Can you work these out from the model? Positions are in its coordinate system, mm. A direction names the side the tool comes from. Round coordinates to 2 decimals unless told otherwise and drop trailing zeros. Write each loop counter-clockwise with the first axis right and the second up, starting at its lowest first coordinate (ties: lowest second). Pieces come first, ordered by that corner, then holes. Notation, with made-up numbers: (32.5, 19) -> (40.5, 19) arc R23 ccw to (40.5, 45) -> close; hole circle Ø8 at (26, -16). An arc over 180 degrees is marked (long way). Use CSV: the item, a comma, the result in double quotes.
```python
from build123d import *

# Parameters (mm, degrees)
SKETCH1_W                = 150.2
SKETCH1_H                = 64
BOSS_EXTRUDE1_DEPTH      = 6
FILLET1_R                = 5
BOSS_EXTRUDE2_DEPTH      = 40
BOSS_EXTRUDE2_DEPTH_BACK = 10
SKETCH2_W                = 60
SKETCH2_H                = 6
FILLET2_R                = 5
SKETCH3_R                = 40
BOSS_EXTRUDE4_DEPTH      = 6
FILLET4_R                = 5
SKETCH4_R                = 1.55
CUT_EXTRUDE1_DEPTH       = 167.673453195
CUT_EXTRUDE2_START       = -10
CUT_EXTRUDE2_DEPTH       = 10
FILLET5_R                = 5
SKETCH6_R                = 1.5
CUT_EXTRUDE3_DEPTH       = 167.673453195
SKETCH7_R                = 1.5
CUT_EXTRUDE4_DEPTH       = 167.673453195
SKETCH9_R                = 3.2
CUT_EXTRUDE5_DEPTH       = 3


with BuildPart() as part:
    # Sketch1 → Boss-Extrude1 (new body)
    with BuildSketch(Plane.XY):
        with Locations((75.1, 32)):
            Rectangle(SKETCH1_W, SKETCH1_H)
    extrude(amount=BOSS_EXTRUDE1_DEPTH)

    # Fillet1
    fillet1_edges = [part.edges().sort_by_distance(p)[0] for p in [
        (0, 64, 3),
        (150.2, 64, 3),
        (150.2, 0, 3),
        (0, 0, 3),
    ]]
    fillet(fillet1_edges, radius=FILLET1_R)

    # Sketch2 → Boss-Extrude2 (add, two sides: drawn at the far end of the back side and taken through both)
    with BuildSketch(Plane.XZ.offset(-BOSS_EXTRUDE2_DEPTH_BACK)):
        with Locations((30, 3)):
            Rectangle(SKETCH2_W, SKETCH2_H)
    extrude(amount=BOSS_EXTRUDE2_DEPTH + BOSS_EXTRUDE2_DEPTH_BACK)

    # Fillet2
    fillet2_edges = [part.edges().sort_by_distance(p)[0] for p in [
        (0, -40, 3),
        (60, -40, 3),
    ]]
    fillet(fillet2_edges, radius=FILLET2_R)

    # Sketch3 → Boss-Extrude4 (add)
    with BuildSketch(Plane.XY.offset(6)):
        with Locations((75.1, 32)):
            Circle(SKETCH3_R)
    extrude(amount=-BOSS_EXTRUDE4_DEPTH)

    # Fillet4
    fillet4_edges = [part.edges().sort_by_distance(p)[0] for p in [
        (60, -5.040383367, 3),
        (99.1, 0, 3),
        (99.1, 64, 3),
        (51.1, 64, 3),
    ]]
    fillet(fillet4_edges, radius=FILLET4_R)

    # Sketch4 → Cut-Extrude1 (cut, through all)
    with BuildSketch(Plane.XY.offset(6)):
        with Locations((75.1, 41.525)):
            Circle(SKETCH4_R)
        with Locations((83.348891971, 36.7625)):
            Circle(SKETCH4_R)
        with Locations((83.348891971, 27.2375)):
            Circle(SKETCH4_R)
        with Locations((75.1, 22.475)):
            Circle(SKETCH4_R)
        with Locations((66.851108029, 27.2375)):
            Circle(SKETCH4_R)
        with Locations((66.851108029, 36.7625)):
            Circle(SKETCH4_R)
    extrude(amount=-CUT_EXTRUDE1_DEPTH, mode=Mode.SUBTRACT)

    # Sketch5 → Cut-Extrude2 (cut)
    with BuildSketch(Plane(origin=(0, 0, 0), x_dir=(-1, 0, 0), z_dir=(0, 0, -1)).offset(CUT_EXTRUDE2_START)):
        with BuildLine():
            Line((0, 0), (-51.1, 0))
            ThreePointArc((-51.1, 0), (-58.245869166, -4.275863516), (-66.122222222, -6.979475448))
            ThreePointArc((-66.122222222, -6.979475448), (-61.886409718, -7.939678347), (-60, -11.851909879))
            Line((-60, -11.851909879), (-60, -35))
            ThreePointArc((-60, -35), (-58.535533906, -38.535533906), (-55, -40))
            Line((-55, -40), (-5, -40))
            ThreePointArc((-5, -40), (-1.464466094, -38.535533906), (0, -35))
            Line((0, -35), (0, 0))
        make_face()
    extrude(amount=CUT_EXTRUDE2_DEPTH, mode=Mode.SUBTRACT)

    # Fillet5
    fillet5_edges = [part.edges().sort_by_distance(p)[0] for p in [
        (0, 0, 3),
    ]]
    fillet(fillet5_edges, radius=FILLET5_R)

    # Sketch6 → Cut-Extrude3 (cut, through all)
    with BuildSketch(Plane.XY.offset(6)):
        with Locations((15, 11)):
            Circle(SKETCH6_R)
        with Locations((15, 53)):
            Circle(SKETCH6_R)
    extrude(amount=-CUT_EXTRUDE3_DEPTH, mode=Mode.SUBTRACT)

    # Sketch7 → Cut-Extrude4 (cut, through all)
    with BuildSketch(Plane.XY.offset(6)):
        with Locations((67, 53)):
            Circle(SKETCH7_R)
        with Locations((67, 11)):
            Circle(SKETCH7_R)
    extrude(amount=-CUT_EXTRUDE4_DEPTH, mode=Mode.SUBTRACT)

    # Sketch9 → Cut-Extrude5 (cut)
    with BuildSketch(Plane.XY.offset(6)):
        with Locations((15, 53)):
            Circle(SKETCH9_R)
        with Locations((67, 53)):
            Circle(SKETCH9_R)
        with Locations((15, 11)):
            Circle(SKETCH9_R)
        with Locations((67, 11)):
            Circle(SKETCH9_R)
    extrude(amount=-CUT_EXTRUDE5_DEPTH, mode=Mode.SUBTRACT)


solid = part.part
```
Q1. If we mould it in two halves opening along X, with no side actions, what happens to faces 1 (the face through (74.898, 43.062, 3.042)), 2 (the face through (148.7, 1.43, 3.04)), 3 (the face through (123, 0, 3))? For each: released by +X, released by -X, zero draft, split by the parting line, or undercut.
Resolved:
face 1,"undercut"
face 2,"released by +X"
face 3,"zero draft"
Q2. Suppose I cut it at D-D (y = -2.5). Write out the boundary of the cut face in (x, z), and give its area (3 significant figures).
Resolved:
outline,"(54.86, 0) -> (95.34, 0) -> (95.34, 6) -> (54.86, 6) -> close"
area,"243 mm^2"
Q3. Will these pins go through, and if not, where does the flat tip stop? P1, Ø1.9, axis at x = 14.5, y = 10.5, coming from the +Z side; P2, Ø1.8, axis at x = 27, z = 2, coming from the -Y side; P3, Ø4, axis at x = 83.35, y = 27.24, coming from the +Z side; P4, Ø2.5, axis at x = 83.35, y = 36.76, coming from the +Z side.
Resolved:
P1,"stops at z = 3"
P2,"stops at y = 0"
P3,"stops at z = 6"
P4,"passes through"
Q4. On a 3-axis mill with a long thin cutter (end or side, diameter ignored), from which of +Z, -Z, +X, -X, +Y, -Y can I reach the whole of each face in a straight line? I mean faces 4 (the face through (14.583, 56.173, 4.521)), 5 (the face through (13.5, 11.07, 1.52)), 6 (the face through (28, 0, 3)), 7 (the face through (27, 64, 3)). Say none if no direction works.
Resolved:
face 4,"+Z"
face 5,"+Z, -Z"
face 6,"+Z, -Z, -X, -Y"
face 7,"+Z, -Z, -X, +Y"
Q5. Suppose I cut it at C-C (x = 43.5). Write out the boundary of the cut face in (y, z).
Resolved:
outline,"(0, 0) -> (64, 0) -> (64, 6) -> (0, 6) -> close"
Q6. Please list where these lines run through material, in increasing order: probe 1 along Y at (x, z) = (75, 0.8); probe 2 along Y at (x, z) = (67, 1.3); probe 3 along Y at (x, z) = (67, 5.05).
Resolved:
probe 1,"y = -8 to 20.93, 24.02 to 39.98, 43.07 to 72"
probe 2,"y = -7.17 to 9.5, 12.5 to 25.69, 28.78 to 35.22, 38.31 to 51.5, 54.5 to 71.17"
probe 3,"y = -7.17 to 7.8, 14.2 to 25.69, 28.78 to 35.22, 38.31 to 49.8, 56.2 to 71.17"
Q7. Suppose I cut it at B-B (y = 11). Write out the boundary of the cut face in (x, z), and give its area (3 significant figures).
Resolved:
outline,"(0, 0) -> (13.5, 0) -> (13.5, 3) -> (11.8, 3) -> (11.8, 6) -> (0, 6) -> close; (16.5, 0) -> (65.5, 0) -> (65.5, 3) -> (63.8, 3) -> (63.8, 6) -> (18.2, 6) -> (18.2, 3) -> (16.5, 3) -> close; (68.5, 0) -> (150.2, 0) -> (150.2, 6) -> (70.2, 6) -> (70.2, 3) -> (68.5, 3) -> close"
area,"845 mm^2"
Q8. Suppose I cut it at A-A (x = 75.1). Write out the boundary of the cut face in (y, z) (3 decimals).
Resolved:
outline,"(-8, 0) -> (20.925, 0) -> (20.925, 6) -> (-8, 6) -> close; (24.025, 0) -> (39.975, 0) -> (39.975, 6) -> (24.025, 6) -> close; (43.075, 0) -> (72, 0) -> (72, 6) -> (43.075, 6) -> close"
